The model under review builds one solid part; all positions refer to its coordinate system, in mm. Face numbers are marked on the shaded views. A direction names the side the tool comes from. Give positions to 0.01 mm unless a question says otherwise; leave off trailing zeros. Order: outer loops, then holes, each group sorted by start corner. A loop starts at its lowest first (then second) coordinate and runs counter-clockwise, first axis right, second up. Notation, with made-up numbers: (82.25, 15.5) - (93.25, 15.5) arc R35 ccw to (93.25, 51.5) - close; hole circle Ø7 at (57, 43.25). An arc over 180 degrees is marked (long way). Use a Markdown table: item, result. Add a question column.
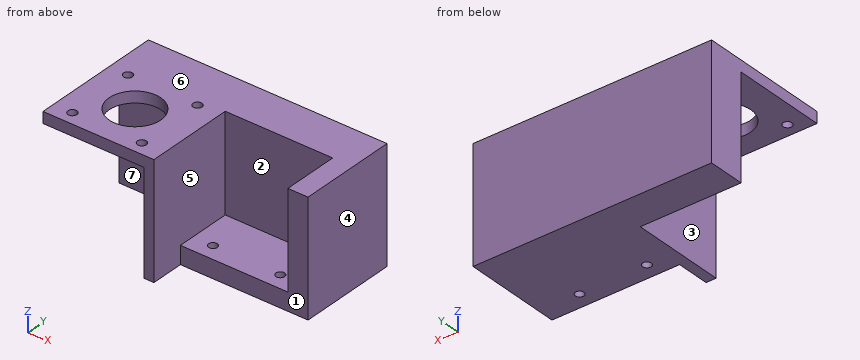
```python
from build123d import *

# Parameters (mm, degrees)
SKETCH1_W            = 48
SKETCH1_H            = 53
BOSS_EXTRUDE1_DEPTH  = 10
SKETCH2_W            = 48
SKETCH2_H            = 5.616325
BOSS_EXTRUDE2_DEPTH  = 33.1917878
SKETCH4_W            = 4
SKETCH4_H            = 10
BOSS_EXTRUDE4_DEPTH  = 40
SKETCH5_W            = 48
SKETCH5_H            = 10.8609375
BOSS_EXTRUDE5_DEPTH  = 23.1917878
SKETCH6_W            = 48
SKETCH6_H            = 5
BOSS_EXTRUDE6_DEPTH  = 42.3
SKETCH7_W            = 12.8082122
SKETCH7_H            = 16.4772625
BOSS_EXTRUDE7_DEPTH  = 48
CUT_EXTRUDE1_REACH   = 84.426
SKETCH8_R            = 11.5
SKETCH8_R_2          = 2
FILLET1_R            = 10
FILLET2_R            = 4
SKETCH9_W            = 5
SKETCH9_H            = 16.4772625
BOSS_EXTRUDE9_DEPTH  = 48
CUT_EXTRUDE2_DEPTH   = 88.252507127
SKETCH11_W           = 51
SKETCH11_H           = 16.4772625
BOSS_EXTRUDE10_DEPTH = 49.45
BOSS_EXTRUDE11_DEPTH = 46
SKETCH16_W           = 47.95
SKETCH16_H           = 51
BOSS_EXTRUDE14_DEPTH = 2.55
SKETCH14_W           = 5
SKETCH14_H           = 42.3
BOSS_EXTRUDE13_DEPTH = 1.5
SKETCH17_W           = 51
SKETCH17_H           = 19.0272625
BOSS_EXTRUDE15_DEPTH = 9
BOSS_EXTRUDE16_DEPTH = 25
SKETCH19_R           = 1.9304
CUT_EXTRUDE3_DEPTH   = 125.404890183


with BuildPart() as part:
    # Sketch1 → Boss-Extrude1 (new body)
    with BuildSketch(Plane.XY):
        with Locations((24, 26.5)):
            Rectangle(SKETCH1_W, SKETCH1_H)
    extrude(amount=BOSS_EXTRUDE1_DEPTH)

    # Sketch2 → Boss-Extrude2 (add)
    with BuildSketch(Plane(origin=(0, 0, 0), x_dir=(-1, 0, 0), z_dir=(0, 0, -1))):
        with Locations((-24, -2.8081625)):
            Rectangle(SKETCH2_W, SKETCH2_H)
    extrude(amount=-BOSS_EXTRUDE2_DEPTH)

    # Sketch4 → Boss-Extrude4 (add)
    with BuildSketch(Plane.XY.offset(10)):
        with Locations((2, 48)):
            Rectangle(SKETCH4_W, SKETCH4_H)
        with Locations((46, 48)):
            Rectangle(SKETCH4_W, SKETCH4_H)
    extrude(amount=BOSS_EXTRUDE4_DEPTH)

    # Sketch5 → Boss-Extrude5 (add)
    with BuildSketch(Plane.XY.offset(10)):
        with Locations((24, 5.43046875)):
            Rectangle(SKETCH5_W, SKETCH5_H)
    extrude(amount=BOSS_EXTRUDE5_DEPTH)

    # Sketch6 → Boss-Extrude6 (add)
    with BuildSketch(Plane.XZ.offset(5.616325)):
        with Locations((24, 30.6917878)):
            Rectangle(SKETCH6_W, SKETCH6_H)
    extrude(amount=BOSS_EXTRUDE6_DEPTH)

    # Sketch7 → Boss-Extrude7 (add)
    with BuildSketch(Plane.ZY):
        with Locations((-6.4041061, 2.62230625)):
            Rectangle(SKETCH7_W, SKETCH7_H)
    extrude(amount=-BOSS_EXTRUDE7_DEPTH)

    # Sketch8 → Cut-Extrude1 (cut, up to next)
    with BuildSketch(Plane(origin=(0, 0, 28.1917878), x_dir=(-1, 0, 0), z_dir=(0, 0, -1)), mode=Mode.PRIVATE) as cut_extrude1_sk1:
        with Locations((-24, -26.616325)):
            Circle(SKETCH8_R)
    cut_extrude1_tool1 = extrude(cut_extrude1_sk1.sketch, amount=-CUT_EXTRUDE1_REACH, mode=Mode.PRIVATE) & part.part
    # Sketch8 → Cut-Extrude1 (cut, up to next)
    with BuildSketch(Plane(origin=(0, 0, 28.1917878), x_dir=(-1, 0, 0), z_dir=(0, 0, -1)), mode=Mode.PRIVATE) as cut_extrude1_sk2:
        with Locations((-39.5, -11.116325)):
            Circle(SKETCH8_R_2)
    cut_extrude1_tool2 = extrude(cut_extrude1_sk2.sketch, amount=-CUT_EXTRUDE1_REACH, mode=Mode.PRIVATE) & part.part
    # Sketch8 → Cut-Extrude1 (cut, up to next)
    with BuildSketch(Plane(origin=(0, 0, 28.1917878), x_dir=(-1, 0, 0), z_dir=(0, 0, -1)), mode=Mode.PRIVATE) as cut_extrude1_sk3:
        with Locations((-39.5, -42.116325)):
            Circle(SKETCH8_R_2)
    cut_extrude1_tool3 = extrude(cut_extrude1_sk3.sketch, amount=-CUT_EXTRUDE1_REACH, mode=Mode.PRIVATE) & part.part
    # Sketch8 → Cut-Extrude1 (cut, up to next)
    with BuildSketch(Plane(origin=(0, 0, 28.1917878), x_dir=(-1, 0, 0), z_dir=(0, 0, -1)), mode=Mode.PRIVATE) as cut_extrude1_sk4:
        with Locations((-8.5, -11.116325)):
            Circle(SKETCH8_R_2)
    cut_extrude1_tool4 = extrude(cut_extrude1_sk4.sketch, amount=-CUT_EXTRUDE1_REACH, mode=Mode.PRIVATE) & part.part
    # Sketch8 → Cut-Extrude1 (cut, up to next)
    with BuildSketch(Plane(origin=(0, 0, 28.1917878), x_dir=(-1, 0, 0), z_dir=(0, 0, -1)), mode=Mode.PRIVATE) as cut_extrude1_sk5:
        with Locations((-8.5, -42.116325)):
            Circle(SKETCH8_R_2)
    cut_extrude1_tool5 = extrude(cut_extrude1_sk5.sketch, amount=-CUT_EXTRUDE1_REACH, mode=Mode.PRIVATE) & part.part
    add(cut_extrude1_tool1.solids().sort_by_distance((24, -26.616325, 28.191788))[0], mode=Mode.SUBTRACT)
    add(cut_extrude1_tool2.solids().sort_by_distance((39.5, -11.116325, 28.191788))[0], mode=Mode.SUBTRACT)
    add(cut_extrude1_tool3.solids().sort_by_distance((39.5, -42.116325, 28.191788))[0], mode=Mode.SUBTRACT)
    add(cut_extrude1_tool4.solids().sort_by_distance((8.5, -11.116325, 28.191788))[0], mode=Mode.SUBTRACT)
    add(cut_extrude1_tool5.solids().sort_by_distance((8.5, -42.116325, 28.191788))[0], mode=Mode.SUBTRACT)

    # Fillet1
    fillet1_edges = [part.edges().sort_by_distance(p)[0] for p in [
        (24, 10.8609375, 0),
    ]]
    fillet(fillet1_edges, radius=FILLET1_R)

    # Fillet2
    fillet2_edges = [part.edges().sort_by_distance(p)[0] for p in [
        (2, 43, 10),
        (46, 43, 10),
    ]]
    fillet(fillet2_edges, radius=FILLET2_R)

    # Sketch9 → Boss-Extrude9 (add)
    with BuildSketch(Plane(origin=(48, 0, 0), x_dir=(0, 0, -1), z_dir=(1, 0, 0))):
        with Locations((15.3082122, 2.62230625)):
            Rectangle(SKETCH9_W, SKETCH9_H)
    extrude(amount=-BOSS_EXTRUDE9_DEPTH)

    # Sketch10 → Cut-Extrude2 (cut, through all)
    with BuildSketch(Plane(origin=(48, 0, 0), x_dir=(0, 0, -1), z_dir=(1, 0, 0))):
        Polygon((17.8082122, 10.8609375), (-33.1917878, 10.8609375), (-76.887145623, 43.902095521), (-50.794096938, 74.436514195), (27.207463492, 71.105486703), align=None)
    extrude(amount=-CUT_EXTRUDE2_DEPTH, mode=Mode.SUBTRACT)

    # Sketch11 → Boss-Extrude10 (add)
    with BuildSketch(Plane(origin=(48, 0, 0), x_dir=(0, 0, -1), z_dir=(1, 0, 0))):
        with Locations((-7.6917878, 2.62230625)):
            Rectangle(SKETCH11_W, SKETCH11_H)
    extrude(amount=BOSS_EXTRUDE10_DEPTH)

    # Sketch12 → Boss-Extrude11 (add)
    with BuildSketch(Plane(origin=(0, 0, 28.1917878), x_dir=(-1, 0, 0), z_dir=(0, 0, -1))):
        Polygon((-48, -47.916325), (-45, -47.916325), (-45, -5.616325), (-49.5, -5.616325), (-49.5, -47.916325), align=None)
    extrude(amount=BOSS_EXTRUDE11_DEPTH)

    # Sketch16 → Boss-Extrude14 (add)
    with BuildSketch(Plane.XZ.offset(5.616325)):
        with Locations((73.475, 7.6917878)):
            Rectangle(SKETCH16_W, SKETCH16_H)
    extrude(amount=BOSS_EXTRUDE14_DEPTH)

    # Sketch14 → Boss-Extrude13 (add)
    with BuildSketch(Plane(origin=(49.5, 0, 0), x_dir=(0, 0, -1), z_dir=(1, 0, 0))):
        with Locations((-30.6917878, -26.766325)):
            Rectangle(SKETCH14_W, SKETCH14_H)
    extrude(amount=-BOSS_EXTRUDE13_DEPTH)

    # Sketch17 → Boss-Extrude15 (add)
    with BuildSketch(Plane(origin=(97.45, 0, 0), x_dir=(0, 0, -1), z_dir=(1, 0, 0))):
        with Locations((-7.6917878, 1.34730625)):
            Rectangle(SKETCH17_W, SKETCH17_H)
    extrude(amount=BOSS_EXTRUDE15_DEPTH)

    # Sketch18 → Boss-Extrude16 (add)
    with BuildSketch(Plane.XZ.offset(8.166325)):
        Polygon((49.5, -17.8082122), (106.45, -17.8082122), (106.45, -9.8082122), (106.45, 33.1917878), (97.45, 33.1917878), (97.45, -9.8082122), (49.5, -9.8082122), align=None)
    extrude(amount=BOSS_EXTRUDE16_DEPTH)

    # Sketch19 → Cut-Extrude3 (cut, through all)
    with BuildSketch(Plane.XY.offset(-9.8082122)):
        with Locations((58.475, -26.166325)):
            Circle(SKETCH19_R)
        with Locations((88.475, -26.166325)):
            Circle(SKETCH19_R)
    extrude(amount=-CUT_EXTRUDE3_DEPTH, mode=Mode.SUBTRACT)


solid = part.part
```
Q1. Draft analysis for pull direction X (two halves, no side actions). For the marked faces 1, 2, 3 and 4, state which applies: pulls with the +X half, pulls with the -X half, needs draft (parallel to the pull), parting line crosses it, or undercut.
Q2. We need section B-B (y = -30). Write out the cut boundary in (x, z), plus the area to 3 significant figures.
Q3. Machinability: for the marked faces 5, 6 and 7, which of the approach directions +Z, -Z, +X, -X, +Y, -Y give a long, thin tool a straight path to every point of the face, cutting with its end or side? Answer none if there is none.
Q4. We need section A-A (x = 39.5). Write out the cut boundary in (y, z), plus the area to 3 significant figures.
Q5. Wall thickness on probe 1 along Y at (x, z) = (39.5, 29.5); probe 2 along Y at (x, z) = (39, 29); probe 3 along Y at (x, z) = (24, 30): over which ranges is each line inside the solid? List them lowest first.
Q6. We need section D-D (z = 21.5). Write out the cut boundary in (x, y), plus the area to 3 significant figures.
Q7. Clearance check with flat-ended pins moving along their axes: P1, Ø20, axis at y = -19.5, z = 9.5, coming from the -X side; P2, Ø6.5, axis at x = 8.5, y = -11.12, coming from the -Z side; P3, Ø12, axis at x = 85, z = 13.5, coming from the -Y side. State where each tip first meets the part, or that it passes through.
Q8. We need section C-C (x = 24). Write out the cut boundary in (y, z), plus the area to 3 significant figures.
Here are the results:
| question | item | result |
|---|---|---|
| 1 | face 1 | needs draft |
| 1 | face 2 | undercut |
| 1 | face 3 | pulls with the -X half |
| 1 | face 4 | pulls with the +X half |
| 2 | outline | (0, 28.19) - (13.01, 28.19) - (13.01, 33.19) - (0, 33.19) - close; (34.99, 28.19) - (45, 28.19) - (45, -17.81) - (106.45, -17.81) - (106.45, 33.19) - (97.45, 33.19) - (97.45, -9.81) - (49.5, -9.81) - (49.5, 33.19) - (34.99, 33.19) - close |
| 2 | area | 1,190 mm2 |
| 3 | face 5 | +Z, -Y |
| 3 | face 6 | +Z, +X, -X, +Y, -Y |
| 3 | face 7 | -Z, -X, -Y |
| 4 | outline | (-47.92, 28.19) - (-44.12, 28.19) - (-44.12, 33.19) - (-47.92, 33.19) - close; (-40.12, 28.19) - (-13.12, 28.19) - (-13.12, 33.19) - (-40.12, 33.19) - close; (-9.12, 28.19) - (-5.62, 28.19) - (-5.62, -17.81) - (10.86, -17.81) - (10.86, 33.19) - (-9.12, 33.19) - close |
| 4 | area | 1,010 mm2 |
| 5 | probe 1 | -47.92 to -44.12, -40.12 to -13.12, -9.12 to 10.86 |
| 5 | probe 2 | -47.92 to -44.05, -40.18 to -13.05, -9.18 to 10.86 |
| 5 | probe 3 | -47.92 to -38.12, -15.12 to 10.86 |
| 6 | outline | (0, -5.62) - (45, -5.62) - (45, -47.92) - (49.5, -47.92) - (49.5, -8.17) - (97.45, -8.17) - (97.45, -33.17) - (106.45, -33.17) - (106.45, 10.86) - (0, 10.86) - close |
| 6 | area | 2,310 mm2 |
| 7 | P1 | x = 45 |
| 7 | P2 | z = 28.19 |
| 7 | P3 | y = -8.17 |
| 8 | outline | (-47.92, 28.19) - (-38.12, 28.19) - (-38.12, 33.19) - (-47.92, 33.19) - close; (-15.12, 28.19) - (-5.62, 28.19) - (-5.62, -17.81) - (10.86, -17.81) - (10.86, 33.19) - (-15.12, 33.19) - close |
| 8 | area | 937 mm2 |
